Design review of the part built by this model. Coordinates are the model's own, in mm. Face numbers are marked on the shaded views. Coordinates: 2 decimals unless noted, no trailing zeros. Loops run counter-clockwise (first coordinate to the right, second up) from the corner with the lowest first, then second, coordinate; pieces in that order, holes last. Notation, with made-up numbers: (21.5, 60) -> (33.5, 60) arc R18 ccw to (33.5, 77) -> close; hole circle Ø10 at (53, 78). An arc over 180 degrees is marked (long way). Use a Markdown table: item, result. Add a question column.
Q1. For probe 1 along X at (y, z) = (103.5, 3.5); probe 2 along Y at (x, z) = (57, 1.2); probe 3 along Y at (x, z) = (57, 5.25), list the stretches that pass through material, from the lowest coordinate up.
Q2. Take a section at D-D on x = 13.5. Write out the cut boundary in (y, z), plus the area to 3 significant figures.
Q3. Take a section at C-C on z = 4.75. Write out the cut boundary in (x, y), plus the area to 3 significant figures.
Q4. Clearance check with flat-ended pins moving along their axes: pin 1 Ø12 at (x, y) = (57.5, 21.5) entering from +Z; pin 2 Ø7 at (x, y) = (102.962, 102.962) entering from +Z. State where each tip first meets the part, or that it passes through.
Q5. Take a section at A-A on x = 57. Write out the cut boundary in (y, z).
Q6. Draft analysis for pull direction X (two halves, no side actions). For the marked faces 1 and 2, state which applies: pulls with the +X half, pulls with the -X half, needs draft (parallel to the pull), parting line crosses it, or undercut.
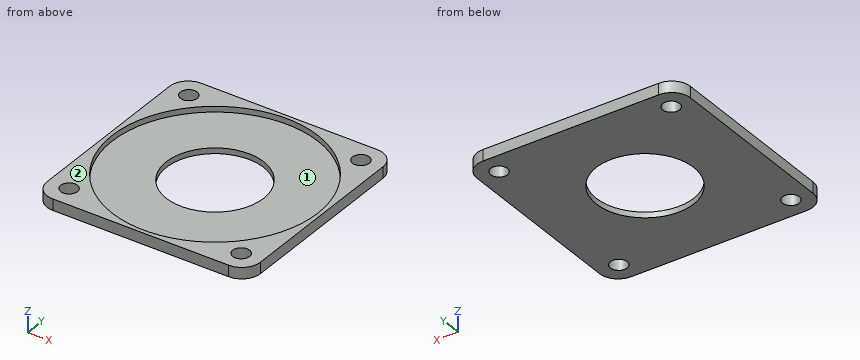
Autodesk Inventor part; units mm, degrees
ref_plane "YZ Plane" through (0, 0, 0) normal (1, 0, 0) x (0, 1, 0)
ref_plane "XZ Plane" through (0, 0, 0) normal (0, 1, 0) x (-1, 0, 0)
ref_plane "XY Plane" through (0, 0, 0) normal (0, 0, 1) x (1, 0, 0)
sketch "Sketch1" plane through (0, 0, 0) normal (0, 0, 1) x (1, 0, 0)
  line L0 (0, 0) -> (114, 0)
  line L1 (114, 0) -> (114, 114)
  line L2 (114, 114) -> (0, 114)
  line L3 (0, 114) -> (0, 0)
  dimension "d0" = 114
  dimension "d1" = 114
extrude "Extrusion1" add sketch "Sketch1" along normal blind 6
sketch "Sketch2" plane through (0, 0, 6) normal (0, 0, 1) x (1, 0, 0)
  circle A0 centre (57, 57) radius 55
  line L0 (0, 114) -> (0, 0)
  line L1 (0, 0) -> (114, 0)
  dimension "d4" = 110
  dimension "d5" = 57
  dimension "d6" = 57
extrude "Extrusion2" cut sketch "Sketch2" against normal blind 3
fillet "Fillet1" radius 10 1 edges at (0, 114, 3)
fillet "Fillet2" radius 10 3 edges at (114, 114, 3) (114, 0, 3) (0, 0, 3)
sketch "Sketch3" plane through (0, 0, 6) normal (0, 0, 1) x (1, 0, 0)
  circle A0 centre (11.038, 11.038) radius 4.5
  line L0 (10, 0) -> (104, 0)
  line L1 (0, 104) -> (0, 10)
  circle A1 centre (11.038, 102.962) radius 4.5
  circle A2 centre (102.962, 102.962) radius 4.5
  circle A3 centre (102.962, 11.038) radius 4.5
  line L2 (104, 114) -> (10, 114)
  line L3 (114, 10) -> (114, 104)
  point P0 (0, 0)
  dimension "d11" = 9
  dimension "d12" = 11.038
  dimension "d13" = 11.038
  dimension "d14" = 9
  dimension "d15" = 9
  dimension "d16" = 9
  dimension "d17" = 11.038
  dimension "d18" = 11.038
  dimension "d19" = 11.038
  dimension "d20" = 11.038
  dimension "d21" = 11.038
  dimension "d22" = 11.038
extrude "Extrusion3" cut sketch "Sketch3" against normal blind 6
sketch "Sketch4" plane through (57, 57, 3) normal (0, 0, 1) x (1, 0, 0)
  circle A0 centre (0, 0) radius 26
  line L0 (-57, 47) -> (-57, -47)
  line L1 (-47, -57) -> (47, -57)
  point P0 (-57, -57)
  point P1 (0, -57)
  dimension "d25" = 52
  dimension "d26" = 57
  dimension "d27" = 57
extrude "Extrusion4" cut sketch "Sketch4" against normal blind 10
equation "\"d6\" = d5"
equation "\"d13\" = d12"
equation "\"d17\" = d12"
equation "\"d18\" = d13"
equation "\"d19\" = d18"
equation "\"d20\" = d18"
equation "\"d21\" = d19"
equation "\"d22\" = d21"
properties part number "BackPlate"
Answer list:
| question | item | result |
|---|---|---|
| 1 | probe 1 | 0 to 6.57, 15.51 to 27.63, 86.37 to 98.49, 107.43 to 114 |
| 1 | probe 2 | 0 to 31, 83 to 114 |
| 1 | probe 3 | 0 to 2, 112 to 114 |
| 2 | outline | (0, 0) -> (7.27, 0) -> (7.27, 6) -> (0, 6) -> close; (14.8, 0) -> (99.2, 0) -> (99.2, 6) -> (90.66, 6) -> (90.66, 3) -> (23.34, 3) -> (23.34, 6) -> (14.8, 6) -> close; (106.73, 0) -> (114, 0) -> (114, 6) -> (106.73, 6) -> close |
| 2 | area | 392 mm² |
| 3 | outline | (0, 10) arc R10 ccw to (10, 0) -> (104, 0) arc R10 ccw to (114, 10) -> (114, 104) arc R10 ccw to (104, 114) -> (10, 114) arc R10 ccw to (0, 104) -> close; hole circle Ø110 at (57, 57); hole circle Ø9 at (11.04, 11.04); hole circle Ø9 at (11.04, 102.96); hole circle Ø9 at (102.96, 11.04); hole circle Ø9 at (102.96, 102.96) |
| 3 | area | 3,150 mm² |
| 4 | pin 1 | z = 3 |
| 4 | pin 2 | through |
| 5 | outline | (0, 0) -> (31, 0) -> (31, 3) -> (2, 3) -> (2, 6) -> (0, 6) -> close; (83, 0) -> (114, 0) -> (114, 6) -> (112, 6) -> (112, 3) -> (83, 3) -> close |
| 6 | face 1 | undercut |
| 6 | face 2 | needs draft |
